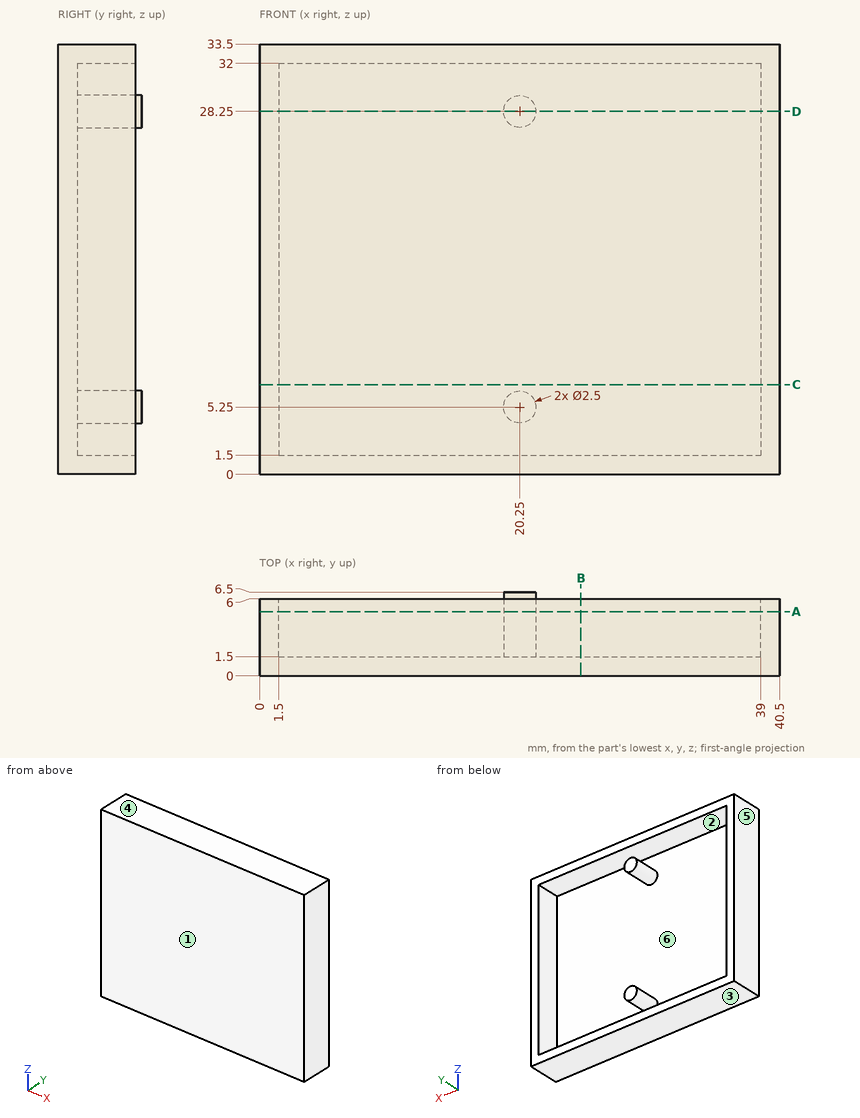
Drawing for the job (mm, zero at the part's lowest x, y, z). A direction names the side the tool comes from. Round coordinates to 2 decimals unless told otherwise and drop trailing zeros. Write each loop counter-clockwise with the first axis right and the second up, starting at its lowest first coordinate (ties: lowest second). Pieces come first, ordered by that corner, then holes. Notation, with made-up numbers: (-30.5, 57) - (-17.5, 57) arc R12 cw to (-17.5, 61) - close; hole circle Ø2 at (34, -39). An arc over 180 degrees is marked (long way). Use CSV: the item, a comma, the result in double quotes.
(1) Wall check: line 1 (Z direction, x = 7, y = 3); line 2 (X direction, y = 2, z = 10); line 3 (Y direction, x = 10.5, z = 11.5). Give the ranges that are in metal, low to high.
Response:
line 1,"0 to 1.5, 32 to 33.5"
line 2,"0 to 1.5, 39 to 40.5"
line 3,"0 to 1.5"
(2) Band-saw the part on C-C (z = 7). Write the cut outline in (x, y).
Response:
outline,"(0, 0) - (40.5, 0) - (40.5, 6) - (39, 6) - (39, 1.5) - (1.5, 1.5) - (1.5, 6) - (0, 6) - close"
(3) Pin check, flat tips, straight feed: P1, Ø1.5, axis at x = 31, z = 15, coming from the +Y side; P2, Ø10, axis at x = 29, z = 29, coming from the +Y side. Stop position of each tip, or through.
Response:
P1,"y = 1.5"
P2,"y = 6"
(4) Band-saw the part on D-D (z = 28.25). Write the cut outline in (x, y), plus the area to 4 significant figures.
Response:
outline,"(0, 0) - (40.5, 0) - (40.5, 6) - (39, 6) - (39, 1.5) - (21.5, 1.5) - (21.5, 6.5) - (19, 6.5) - (19, 1.5) - (1.5, 1.5) - (1.5, 6) - (0, 6) - close"
area,"86.75 mm²"
(5) Band-saw the part on B-B (x = 25). Write the cut outline in (y, z), plus the area to 4 significant figures.
Response:
outline,"(0, 0) - (6, 0) - (6, 1.5) - (1.5, 1.5) - (1.5, 32) - (6, 32) - (6, 33.5) - (0, 33.5) - close"
area,"63.75 mm²"
(6) Band-saw the part on A-A (y = 5). Write the cut outline in (x, z).
Response:
outline,"(0, 0) - (40.5, 0) - (40.5, 33.5) - (0, 33.5) - close; circle Ø2.5 at (20.25, 5.25); circle Ø2.5 at (20.25, 28.25); hole (1.5, 1.5) - (39, 1.5) - (39, 32) - (1.5, 32) - close"
(7) Mould opens along Z. For the marked faces 1, 2, 3 and 4 say: pulls with the +Z half, pulls with the -Z half, needs draft (parallel to the pull), parting line crosses it, or undercut.
Response:
face 1,"needs draft"
face 2,"undercut"
face 3,"pulls with the -Z half"
face 4,"pulls with the +Z half"
(8) 3-axis set-ups, long thin cutter, end or side, ignore diameter. For the marked faces 5 and 6: which of +Z, -Z, +X, -X, +Y, -Y reach the whole face in a straight line?
Response:
face 5,"+Z, -Z, -X, +Y, -Y"
face 6,"+Y"
